Autodesk Inventor part; units mm, degrees
ref_plane "YZ Plane" through (0, 0, 0) normal (1, 0, 0) x (0, 1, 0)
ref_plane "XZ Plane" through (0, 0, 0) normal (0, 1, 0) x (-1, 0, 0)
ref_plane "XY Plane" through (0, 0, 0) normal (0, 0, 1) x (1, 0, 0)
sketch "Sketch1" plane through (0, 0, 0) normal (0, 0, 1) x (1, 0, 0)
  line L0 (-38.5, -31.5) -> (38.5, -31.5)
  line L1 (38.5, -31.5) -> (38.5, 31.5)
  line L2 (38.5, 31.5) -> (-38.5, 31.5)
  line L3 (-38.5, 31.5) -> (-38.5, -31.5)
  line L4 (-38.5, -31.5) -> (38.5, 31.5) construction
  line L5 (38.5, -31.5) -> (-38.5, 31.5) construction
  point P0 (0, 0)
  dimension "d0" = 77
  dimension "d1" = 63
extrude "Extrusion1" add sketch "Sketch1" along normal blind 3
sketch "Sketch2" plane through (0, 0, 3) normal (0, 0, 1) x (1, 0, 0)
  line L0 (-38.5, 31.5) -> (-38.5, -31.5)
  line L1 (-38.5, -31.5) -> (-35.5, -31.5)
  line L2 (-35.5, -31.5) -> (-35.5, -1.5)
  line L3 (-35.5, -1.5) -> (-38.5, -1.5)
  line L4 (-38.5, -1.5) -> (-38.5, -31.5)
  line L5 (-38.5, -31.5) -> (38.5, -31.5)
  line L6 (38.5, -31.5) -> (35.5, -31.5)
  line L7 (35.5, -31.5) -> (35.5, -1.5)
  line L8 (35.5, -1.5) -> (38.5, -1.5)
  line L9 (38.5, -1.5) -> (38.5, -31.5)
  line L10 (-18.5, -31.5) -> (1.5, -31.5)
  line L11 (1.5, -31.5) -> (1.5, -28.5)
  line L12 (1.5, -28.5) -> (-18.5, -28.5)
  line L13 (-18.5, -28.5) -> (-18.5, -31.5)
  line L14 (35.5, -31.5) -> (21.5, -31.5)
  line L15 (21.5, -31.5) -> (21.5, -28.5)
  line L16 (21.5, -28.5) -> (35.5, -28.5)
  line L17 (35.5, -28.5) -> (35.5, -31.5)
  point P0 (0, 0)
  dimension "d4" = 3
  dimension "d5" = 30
  dimension "d6" = 3
  dimension "d7" = 30
  dimension "d8" = 20
  dimension "d9" = 3
  dimension "d10" = 20
  dimension "d11" = 3
  dimension "d12" = 20
extrude "Extrusion2" cut sketch "Sketch2" against normal through all
sketch "Sketch3" plane through (0, 0, 3) normal (0, 0, 1) x (1, 0, 0)
  line L0 (38.5, 31.5) -> (-38.5, 31.5)
  line L1 (-18.5, 31.5) -> (1.5, 31.5)
  line L2 (1.5, 31.5) -> (1.5, 28.5)
  line L3 (1.5, 28.5) -> (-18.5, 28.5)
  line L4 (-18.5, 28.5) -> (-18.5, 31.5)
  line L5 (-38.5, 31.5) -> (-38.5, -1.5)
  point P0 (0, 0)
  dimension "d15" = 20
  dimension "d16" = 3
  dimension "d17" = 20
extrude "Extrusion3" cut sketch "Sketch3" against normal blind 3
properties part number "front_left"
CAD build for the part. Positions are in the model's coordinates, mm. A direction names the side the tool comes from. Coordinates: 2 decimals unless noted, no trailing zeros. Order: outer loops, then holes, each group sorted by start corner. A loop starts at its lowest first (then second) coordinate and runs counter-clockwise, first axis right, second up.
(1) Pin check, flat tips, straight feed: pin 1 Ø1.5 at (x, z) = (37, 1) entering from -Y; pin 2 Ø1.5 at (y, z) = (-13.5, 2) entering from +X; pin 3 Ø1.5 at (x, z) = (-13, 1.5) entering from +Y. Stop position of each tip, or through.
Solution:
pin 1: stops at y = -1.5
pin 2: stops at x = 35.5
pin 3: stops at y = 28.5
(2) Which spindle directions (+Z, -Z, +X, -X, +Y, -Y) get a long thin tool onto all of the face, cutting with end or side? Do faces 4 (the face through (1.5, 30, 2)), 5 (the face through (-37, -1.5, 2)), 6 (the face through (35.5, -15, 2)), 7 (the face through (1.5, -30, 2)). Say none if no direction does.
Solution:
face 4: +Z, -Z, +Y
face 5: +Z, -Z, -X, -Y
face 6: +Z, -Z, +X, -Y
face 7: +Z, -Z, -Y
(3) Mould opens along X. For faces 1 (the face through (-1, 0, 0)), 2 (the face through (21.5, -30, 2)), 3 (the face through (-18.5, 30, 2)) say: released by +X, released by -X, zero draft, split by the parting line, or undercut.
Solution:
face 1: zero draft
face 2: released by +X
face 3: undercut
(4) Saw through at B-B, the plane x = 31. Write the cut outline in (y, z), and give its area (3 significant figures).
Solution:
outline: (-28.5, 0) - (31.5, 0) - (31.5, 3) - (-28.5, 3) - close
area: 180 mm2
(5) Saw through at C-C, the plane y = -22.5. Write the cut outline in (x, z).
Solution:
outline: (-35.5, 0) - (35.5, 0) - (35.5, 3) - (-35.5, 3) - close
(6) Drill centre lines: L1, parallel to Y at x = -2.5, z = 1.85; L2, parallel to X at y = -11.5, z = 1.2; L3, parallel to Y at x = 25, z = 1.85. Where is each one in solid material? Low to high.
Solution:
L1: y = -28.5 to 28.5
L2: x = -35.5 to 35.5
L3: y = -28.5 to 31.5
(7) Saw through at A-A, the plane z = 1. Write the cut outline in (x, y).
Solution:
outline: (-38.5, -1.5) - (-35.5, -1.5) - (-35.5, -31.5) - (-18.5, -31.5) - (-18.5, -28.5) - (1.5, -28.5) - (1.5, -31.5) - (21.5, -31.5) - (21.5, -28.5) - (35.5, -28.5) - (35.5, -1.5) - (38.5, -1.5) - (38.5, 31.5) - (1.5, 31.5) - (1.5, 28.5) - (-18.5, 28.5) - (-18.5, 31.5) - (-38.5, 31.5) - close
